from build123d import *

# Parameters (mm, degrees)
F1_R     = 4.7625
F4_DEPTH = 6.35
F6_DEPTH = 4.826
F2_R     = 3.175
F7_DEPTH = 12.7
F9_SIZE2 = 0.762
F9_SIZE  = 0.762
F10_R    = 0.508


# Not quite as in the source:
# - the program builds the solid bodies; features that only make, move or delete a surface that nothing else refers to are left out


with BuildPart() as f4:
    # F1 (on Top) → F4 (new body)
    with BuildSketch(Plane.XY):
        Circle(F1_R)
    extrude(amount=F4_DEPTH)

    # F5 (on face) → F6 (cut)
    with BuildSketch(Plane.XY.offset(6.35)):
        Polygon((2.38125, -1.3748153285), (2.38125, 1.3748153285), (0, 2.749630657), (-2.38125, 1.3748153285), (-2.38125, -1.3748153285), (0, -2.749630657), align=None)
    extrude(amount=-F6_DEPTH, mode=Mode.SUBTRACT)

    # F2 (on Top) → F7 (join)
    with BuildSketch(Plane.XY):
        Circle(F2_R)
    extrude(amount=-F7_DEPTH)

    # F9
    f9_edges = [f4.edges().sort_by_distance(p)[0] for p in [
        (-3.175, 0, -12.7),
    ]]
    chamfer(f9_edges, length=F9_SIZE, length2=F9_SIZE2)

    # F10
    f10_edges = [f4.edges().sort_by_distance(p)[0] for p in [
        (-4.7625, 0, 6.35),
        (-4.7625, 0, 0),
    ]]
    fillet(f10_edges, radius=F10_R)


solid = f4.part
The model under review builds one solid part; all positions refer to its coordinate system, in mm. A direction names the side the tool comes from. Round coordinates to 2 decimals unless told otherwise and drop trailing zeros. Loops run counter-clockwise (first coordinate to the right, second up) from the corner with the lowest first, then second, coordinate; pieces in that order, holes last. Notation, with made-up numbers: (-32, -16) -> (-27, -16) arc R20 ccw to (-27, 5) -> close; hole circle Ø2 at (45, -11). An arc over 180 degrees is marked (long way). Write item = value, one per line. Start each with the question number.
Item 1: Take a section at B-B on z = -7.25. Give the boundary of the cut face in (x, y) (3 decimals), plus the area to 3 significant figures.
Item 2: To check wall thickness, follow L1, parallel to Z at x = 1, y = -1; L2, parallel to X at y = -2.5, z = 5.25; L3, parallel to Z at x = 3.75, y = 2. State the ranges of each line that lie inside material, in increasing order.
Item 3: For faces 4 (the cylindrical face through (-3.78, -2.9, 3.14)), 5 (the cylindrical face through (-0.69, -3.1, -5.89)), 6 (the flat face through (2.381, 0, 4)), list the 3-axis set-ups (+Z, -Z, +X, -X, +Y, -Y) from which the entire face can be reached by the end or side of a thin tool; tool diameter is ignored.
Item 4: Mouldability with a two-part tool opening along Z and no side actions: class faces 1 (the flat face through (1.174, -2.072, 3.971)), 2 (the flat face through (2, -2, 6.35)), 3 (the flat face through (-2, -3, 0)) as released by +Z, released by -Z, zero draft, split by the parting line, or undercut.
Item 5: Insertion check: pin 1 (1.4 mm diameter, centred on x = 1, y = 1, fed in from +Z); pin 2 (3 mm diameter, centred on y = 0.5, z = 4, fed in from +X); pin 3 (1 mm diameter, centred on y = -3, z = -5, fed in from +X); pin 4 (5 mm diameter, centred on x = -2, z = -5, fed in from +Y) (3 decimals). Each pin has a flat end and moves straight along its axis. Give the tip position at first contact, or say it passes through.
Result:
q1.outline = circle Ø6.35 at (0, 0)
q1.area = 31.7 mm²
q2.L1 = -12.7 to 1.52
q2.L2 = -4.05 to -0.43, 0.43 to 4.05
q2.L3 = 0 to 6.35
q3.face_4 = +Z, -Z
q3.face_5 = -Z
q3.face_6 = +Z
q4.face_1 = zero draft
q4.face_2 = released by +Z
q4.face_3 = released by -Z
q5.pin_1 = 1.52
q5.pin_2 = 4.76
q5.pin_3 = 1.96
q5.pin_4 = 3.175
